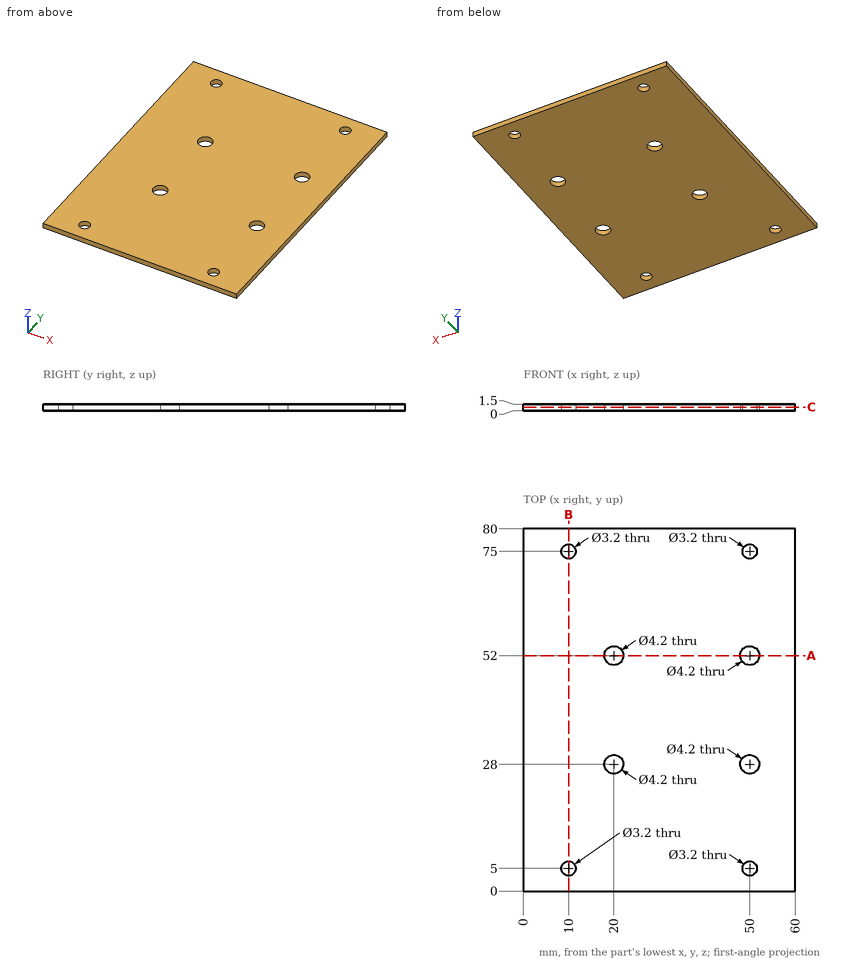
The drawing under review shows one solid part. Ordinate dimensions are in mm from its lowest x, y, z. Give positions to 0.01 mm unless a question says otherwise; leave off trailing zeros. Write each loop counter-clockwise with the first axis right and the second up, starting at its lowest first coordinate (ties: lowest second). Pieces come first, ordered by that corner, then holes. Notation, with made-up numbers: (1, 8.5) - (23, 8.5) arc R15 cw to (23, 27.5) - close; hole circle Ø8 at (-0.5, 80.5). An arc over 180 degrees is marked (long way). Answer in a Markdown table with one row per item. Add a question column.
1. Wall thickness on line 1 along Y through (x, z) = (10, 0.3); line 2 along X through (y, z) = (52, 1.1); line 3 along X through (y, z) = (5, 1.15): over which ranges is each line inside the solid? List them lowest first. Write a range as [from, to].
2. We need section A-A on y = 52. Write out the cut boundary in (x, z).
3. We need section B-B on x = 10. Write out the cut boundary in (y, z).
4. We need section C-C on z = 0.8. State how many separate pieces and enclosed holes the cut face has, then the cut area to 3 significant figures.
Ans:
| question | item | result |
|---|---|---|
| 1 | line 1 | y = [0, 3.4], [6.6, 73.4], [76.6, 80] |
| 1 | line 2 | x = [0, 17.9], [22.1, 47.9], [52.1, 60] |
| 1 | line 3 | x = [0, 8.4], [11.6, 48.4], [51.6, 60] |
| 2 | outline | (0, 0) - (17.9, 0) - (17.9, 1.5) - (0, 1.5) - close; (22.1, 0) - (47.9, 0) - (47.9, 1.5) - (22.1, 1.5) - close; (52.1, 0) - (60, 0) - (60, 1.5) - (52.1, 1.5) - close |
| 3 | outline | (0, 0) - (3.4, 0) - (3.4, 1.5) - (0, 1.5) - close; (6.6, 0) - (73.4, 0) - (73.4, 1.5) - (6.6, 1.5) - close; (76.6, 0) - (80, 0) - (80, 1.5) - (76.6, 1.5) - close |
| 4 | separate pieces | 1 |
| 4 | enclosed holes | 8 |
| 4 | area | 4,710 mm^2 |
